CAD build for the part. Positions are in the model's coordinates, mm. Face numbers are marked on the shaded views. Give positions to 0.01 mm unless a question says otherwise; leave off trailing zeros. Loops run counter-clockwise (first coordinate to the right, second up) from the corner with the lowest first, then second, coordinate; pieces in that order, holes last. Notation, with made-up numbers: (-21, 25.5) -> (14, 25.5) arc R23 ccw to (14, 48.5) -> close; hole circle Ø5 at (38, 39). An arc over 180 degrees is marked (long way). Use one line per item in the form item = value.
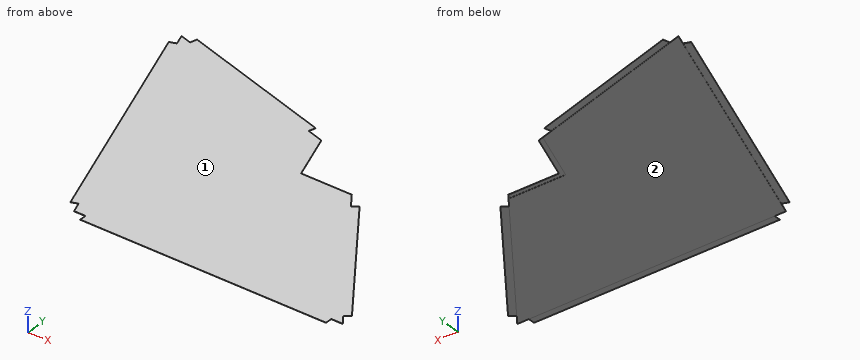
Autodesk Inventor part; units mm, degrees
ref_plane "YZ Plane" through (0, 0, 0) normal (1, 0, 0) x (0, 1, 0)
ref_plane "XZ Plane" through (0, 0, 0) normal (0, 1, 0) x (-1, 0, 0)
ref_plane "XY Plane" through (0, 0, 0) normal (0, 0, 1) x (1, 0, 0)
sketch "Sketch1" plane through (0, 0, 0) normal (0, 0, 1) x (1, 0, 0)
  line L0 (-149.2247, -82.55) -> (149.2253, -82.55)
  line L1 (31.75, 82.55) -> (-31.75, 82.55)
  line L2 (31.75, 82.55) -> (149.2253, -82.55)
  line L3 (-31.75, 82.55) -> (-149.2247, -82.55)
  line L4 (-149.2247, -82.55) -> (-247.0638, 199.4073)
  line L5 (-31.75, 82.55) -> (-52.5668, 142.5409)
  line L6 (-247.0638, 199.4073) -> (-52.5668, 142.5409)
  point P0 (0, 0)
  point P1 (0, 82.55)
  point P2 (-90.4873, 0)
  dimension "d1" = 298.45
  dimension "d2" = 63.5
  dimension "d3" = 165.1
  dimension "d4" = 202.6285
  dimension "d5" = 202.6289
  dimension "d31" = 125.433
  dimension "d32" = 125.433
  dimension "d33" = 54.567
  dimension "d34" = 54.567
  dimension "d35" = 54.57
  dimension "d36" = 298.45
  dimension "d37" = 125.43
  dimension "d38" = 63.5
  dimension "d39" = 202.6397
  dimension "d40" = 54.566
  dimension "d41" = 125.434
extrude "Extrusion2" add sketch "Sketch1" along normal blind 0.127
sketch "Sketch3" plane through (0, 0, 0.127) normal (0, 0, 1) x (1, 0, 0)
  line L0 (31.75, 82.55) -> (-31.75, 82.55)
  line L1 (-31.75, 82.55) -> (31.75, 82.55)
  line L2 (-31.75, 82.55) -> (-28.1358, 87.63)
  line L3 (31.75, 82.55) -> (28.1358, 87.63)
  line L4 (-28.1358, 87.63) -> (28.1358, 87.63)
  line L5 (-31.75, 82.55) -> (-52.5668, 142.5409)
  line L6 (-52.5668, 142.5409) -> (-46.5827, 140.7918)
  line L7 (-46.5827, 140.7918) -> (-28.1358, 87.63)
  line L8 (-149.2247, -82.55) -> (149.2253, -82.55)
  line L9 (-52.5668, 142.5409) -> (-247.0638, 199.4073)
  line L10 (-247.0638, 199.4073) -> (-149.2247, -82.55)
  line L11 (136.5253, -90.17) -> (-136.5247, -90.17)
  line L12 (-247.0638, 199.4073) -> (-149.2247, -82.55)
  line L13 (-160.5869, -73.0498) -> (-250.0993, 184.9111)
  line L14 (-232.7357, 203.1571) -> (-62.6181, 153.4187)
  line L15 (-31.75, 82.55) -> (31.75, 82.55)
  line L16 (149.2253, -82.55) -> (31.75, 82.55)
  line L17 (45.3216, 76.6199) -> (148.0711, -67.7844)
  line L18 (31.75, 82.55) -> (149.2253, -82.55)
  line L19 (-52.5668, 142.5409) -> (-31.75, 82.55)
  line L20 (-46.5827, 140.7918) -> (-28.1358, 87.63)
  line L21 (-28.1358, 87.63) -> (28.1358, 87.63)
  line L22 (-232.7357, 203.1571) -> (-234.8741, 195.8433)
  line L23 (-64.7565, 146.1049) -> (-62.6181, 153.4187)
  line L24 (-250.0993, 184.9111) -> (-242.9004, 187.4091)
  line L25 (-160.5869, -73.0498) -> (-153.388, -70.5518)
  line L26 (-136.5247, -82.55) -> (-136.5247, -90.17)
  line L27 (136.5253, -82.55) -> (136.5253, -90.17)
  line L28 (148.0711, -67.7844) -> (141.8624, -72.2022)
  line L29 (45.3216, 76.6199) -> (39.1129, 72.2022)
  point P0 (0, 0)
  dimension "d45" = 54.57
  dimension "d46" = 5.08
  dimension "d47" = 54.57
  dimension "d48" = 54.57
  dimension "d51" = 5.08
  dimension "d68" = 7.62
  dimension "d84" = 7.62
  dimension "d89" = 90
  dimension "d90" = 12.7
  dimension "d91" = 7.62
  dimension "d93" = 90
  dimension "d94" = 12.7
  dimension "d95" = 12.7
  dimension "d97" = 12.7
  dimension "d98" = 90
  dimension "d99" = 90
  dimension "d100" = 7.62
  dimension "d101" = 12.7
  dimension "d102" = 12.7
  dimension "d103" = 7.62
  dimension "d104" = 7.62
  dimension "d105" = 12.7
  dimension "d106" = 12.7
  dimension "d107" = 7.62
  dimension "d108" = 7.62
  dimension "d109" = 90
extrude "Extrusion4" add sketch "Sketch3" along normal blind 0.127
sketch "Sketch5" plane through (0, 0, 0.254) normal (0, 0, 1) x (1, 0, 0)
  line L0 (31.75, 82.55) -> (-31.75, 82.55)
  line L1 (31.75, 82.55) -> (-31.75, 82.55)
  line L2 (-149.2247, -82.55) -> (149.2253, -82.55)
  line L3 (31.75, 82.55) -> (149.2253, -82.55)
  line L4 (149.2253, -82.55) -> (-149.2247, -82.55)
  line L5 (-242.9004, 187.4091) -> (-149.2247, -82.55)
  line L6 (-149.2247, -82.55) -> (-247.0638, 199.4073)
  line L7 (-247.0638, 199.4073) -> (-52.5668, 142.5409)
  line L8 (-31.75, 82.55) -> (-52.5668, 142.5409)
  line L9 (-52.5668, 142.5409) -> (-31.75, 82.55)
  line L10 (-31.75, 82.55) -> (-28.1358, 87.63)
  line L11 (-31.75, 82.55) -> (-149.2247, -82.55)
properties part number "DELL screen 3D hologram piece"
1. Drill centre lines: line 1 (X direction, y = 73, z = 0.2); line 2 (X direction, y = 81, z = 0.2); line 3 (X direction, y = 26.5, z = 0.2). Where is each one in solid material? Low to high.
Result sheet:
line_1 = -211.27 to 38.55, 40.23 to 47.9
line_2 = -214.04 to 32.85
line_3 = -195.13 to 80.98
2. Cut at C-C, the plane z = 0.2. Write the cut outline in (x, y).
Result sheet:
outline = (-250.1, 184.91) -> (-160.59, -73.05) -> (-153.39, -70.55) -> (-149.22, -82.55) -> (-136.52, -82.55) -> (-136.52, -90.17) -> (136.53, -90.17) -> (136.53, -82.55) -> (149.23, -82.55) -> (141.86, -72.2) -> (148.07, -67.78) -> (45.32, 76.62) -> (39.11, 72.2) -> (31.75, 82.55) -> (28.14, 87.63) -> (-28.14, 87.63) -> (-46.58, 140.79) -> (-52.57, 142.54) -> (-64.76, 146.1) -> (-62.62, 153.42) -> (-232.74, 203.16) -> (-234.87, 195.84) -> (-247.06, 199.41) -> (-242.9, 187.41) -> close
3. Cut at B-B, the plane y = 22. Write the cut outline in (x, z).
Result sheet:
outline = (-193.57, 0.13) -> (-185.5, 0.13) -> (-185.5, 0) -> (74.83, 0) -> (74.83, 0.13) -> (84.19, 0.13) -> (84.19, 0.25) -> (-193.57, 0.25) -> close
4. Drop a flat-ended pin along its axis: P1, Ø8.5, axis at x = -49, y = -86.5, coming from the -Z side. Give the stop position or say it passes through.
Result sheet:
P1 = 0
5. Cut at A-A, the plane x = 5.5. Write the cut outline in (y, z).
Result sheet:
outline = (-90.17, 0.13) -> (-82.55, 0.13) -> (-82.55, 0) -> (82.55, 0) -> (82.55, 0.13) -> (87.63, 0.13) -> (87.63, 0.25) -> (-90.17, 0.25) -> close
6. Mould opens along Z. For the marked faces 1 and 2 say: pulls with the +Z half, pulls with the -Z half, needs draft (parallel to the pull), parting line crosses it, or undercut.
Result sheet:
face_1 = pulls with the +Z half
face_2 = pulls with the -Z half
